Geometry check sheet. Reference: the model listing, model coordinates, mm. Face numbers are marked on the shaded views. A direction names the side the tool comes from. Give positions to 0.01 mm unless a question says otherwise; leave off trailing zeros. Order: outer loops, then holes, each group sorted by start corner. A loop starts at its lowest first (then second) coordinate and runs counter-clockwise, first axis right, second up.
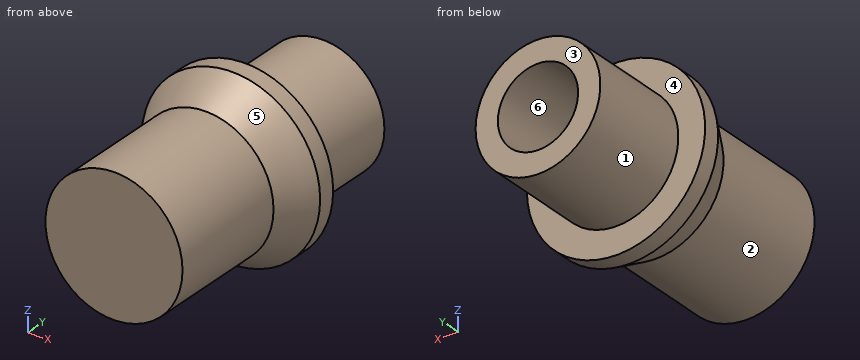
from build123d import *

# Parameters (mm, degrees)
SKETCH1_R           = 3.5
SKETCH1_R_2         = 2.25
BOSS_EXTRUDE1_DEPTH = 6
SKETCH2_R           = 5
BOSS_EXTRUDE2_DEPTH = 1
SKETCH4_R           = 5
BOSS_EXTRUDE4_DEPTH = 2
BOSS_EXTRUDE4_TAPER = 30
SKETCH5_R           = 3.845299462
BOSS_EXTRUDE5_DEPTH = 7


with BuildPart() as part:
    # Sketch1 → Boss-Extrude1 (new body)
    with BuildSketch(Plane(origin=(0, 0, 0), x_dir=(1, 0, 0), z_dir=(0, 1, 0))):
        Circle(SKETCH1_R)
        Circle(SKETCH1_R_2, mode=Mode.SUBTRACT)
    extrude(amount=-BOSS_EXTRUDE1_DEPTH)

    # Sketch2 → Boss-Extrude2 (add)
    with BuildSketch(Plane.XZ.offset(6)):
        Circle(SKETCH2_R)
    extrude(amount=BOSS_EXTRUDE2_DEPTH)

    # Sketch4 → Boss-Extrude4 (add)
    with BuildSketch(Plane.XZ.offset(7)):
        Circle(SKETCH4_R)
    extrude(amount=BOSS_EXTRUDE4_DEPTH, taper=BOSS_EXTRUDE4_TAPER)

    # Sketch5 → Boss-Extrude5 (add)
    with BuildSketch(Plane.XZ.offset(9)):
        Circle(SKETCH5_R)
    extrude(amount=BOSS_EXTRUDE5_DEPTH)


solid = part.part
Item 1: Sectioned sample at C-C (y = -11.25). Enter the section's corners in (x, z), and give its area (3 significant figures).
Reported:
outline: circle Ø7.69 at (0, 0)
area: 46.5 mm2
Item 2: Sectioned sample at B-B (y = -3.25). Enter the section's corners in (x, z).
Reported:
outline: circle Ø7 at (0, 0); hole circle Ø4.5 at (0, 0)
Item 3: Sectioned sample at D-D (y = -7.25). Enter the section's corners in (x, z), and give its area (3 significant figures).
Reported:
outline: circle Ø9.71 at (0, 0)
area: 74.1 mm2
Item 4: Gauge pin test, flat ends, axial feed: pin 1 (1.3 mm diameter, centred on x = 0, z = -1, fed in from +Y); pin 2 (1.5 mm diameter, centred on y = -9.5, z = 0, fed in from -X); pin 3 (1 mm diameter, centred on x = -4, y = -13.5, fed in from +Z). Record the tip position at first contact, or that the pin passes through.
Reported:
pin 1: stops at y = -6
pin 2: stops at x = -3.99
pin 3: stops at z = 1.59
Item 5: Set-up check for the marked faces 1, 2 and 3: record each of +Z, -Z, +X, -X, +Y, -Y from which the full face is reachable in a straight line by a thin tool's end or side.
Reported:
face 1: +Y
face 2: -Y
face 3: +Z, -Z, +X, -X, +Y
Item 6: Draft check along X on the marked faces 4, 5 and 6. Enter one of: released by +X, released by -X, zero draft, split by the parting line, or undercut.
Reported:
face 4: zero draft
face 5: split by the parting line
face 6: undercut
Item 7: Sectioned sample at A-A (x = 0). Enter the section's corners in (y, z).
Reported:
outline: (-16, -3.85) - (-9, -3.85) - (-7, -5) - (-6, -5) - (-6, -3.5) - (0, -3.5) - (0, -2.25) - (-6, -2.25) - (-6, 2.25) - (0, 2.25) - (0, 3.5) - (-6, 3.5) - (-6, 5) - (-7, 5) - (-9, 3.85) - (-16, 3.85) - close
Item 8: Scan lines: L1, parallel to X at y = -3.15, z = 0; L2, parallel to Y at x = 3.5, z = 3. Record each from-to range of solid material in increasing order.
Reported:
L1: x = -3.5 to -2.25, 2.25 to 3.5
L2: y = -7.68 to -6
